Work out the finished part from the listing and answer in its coordinate system (mm). A direction names the side the tool comes from. Round coordinates to 2 decimals unless told otherwise and drop trailing zeros. Loops run counter-clockwise (first coordinate to the right, second up) from the corner with the lowest first, then second, coordinate; pieces in that order, holes last. Notation, with made-up numbers: (17, 53.5) - (74, 53.5) arc R20 ccw to (74, 83.5) - close; hole circle Ø5 at (-19.5, 22). An arc over 180 degrees is marked (long way). Return JSON: item names as keys, results as strings.
Autodesk Inventor part; units mm, degrees
ref_plane "YZ Plane" through (0, 0, 0) normal (1, 0, 0) x (0, 1, 0)
ref_plane "XZ Plane" through (0, 0, 0) normal (0, 1, 0) x (-1, 0, 0)
ref_plane "XY Plane" through (0, 0, 0) normal (0, 0, 1) x (1, 0, 0)
sketch "スケッチ1" plane through (0, 0, 0) normal (0, 0, 1) x (1, 0, 0)
  circle A0 centre (0, 0) radius 27.25
  line L0 (17.5, 17.5) -> (-17.5, 17.5)
  line L1 (-17.5, 17.5) -> (-17.5, -17.5)
  line L2 (-17.5, -17.5) -> (17.5, -17.5)
  line L3 (17.5, -17.5) -> (17.5, 17.5)
  line L4 (17.5, 17.5) -> (-17.5, -17.5) construction
  line L5 (-17.5, 17.5) -> (17.5, -17.5) construction
  line L6 (1, 17.5) -> (-1, 17.5)
  line L7 (-1, 17.5) -> (-1, -17.5)
  line L8 (-1, -17.5) -> (1, -17.5)
  line L9 (1, -17.5) -> (1, 17.5)
  line L10 (1, 17.5) -> (-1, -17.5) construction
  line L11 (-1, 17.5) -> (1, -17.5) construction
  point P0 (1, -17.5)
  point P1 (1, 17.5)
  point P2 (-1, 17.5)
  point P3 (-1, -17.5)
  dimension "d0" = 54.5
  dimension "d6" = 35
  dimension "d107" = 2
  dimension "d108" = 35
extrude "押し出し1" add sketch "スケッチ1" against normal blind 3 contours A0 | L9 L2 L7 L0
sketch "スケッチ2" plane through (0, 0, 0) normal (0, 0, 1) x (1, 0, 0)
  line L0 (0, 42.4511) -> (0, -37.5489)
  line L1 (38.0038, 0) -> (-41.9962, 0)
  line L2 (27.25, 42.0143) -> (27.25, -37.9857)
  circle A0 centre (0, 0) radius 27.25
  line L3 (17.5, 17.5) -> (17.5, -17.5)
  line L4 (19.25, 25) -> (27.25, 25)
  line L5 (27.25, 25) -> (27.25, -25)
  line L6 (27.25, -25) -> (19.25, -25)
  line L7 (19.25, -25) -> (19.25, 25)
  line L8 (19.25, 25) -> (27.25, -25) construction
  line L9 (27.25, 25) -> (19.25, -25) construction
  point P0 (17.5, 0)
  point P1 (23.25, 0)
  point P2 (19.25, 0)
  point P3 (27.25, 0)
  dimension "d13" = 9.75
  dimension "d14" = 8
  dimension "d15" = 50
  dimension "d19" = 54.5
  dimension "d110" = 1.75
extrude "押し出し2" cut sketch "スケッチ2" against normal blind 10 contours L7 L4 L2 A0 | A0 L1 L7 picked at (20.3822, 11.481)
mirror "ミラー1" about plane through (0, 0, 0) normal (1, 0, 0) of "押し出し2"
sketch "スケッチ8" plane through (0, 0, 0) normal (0, 0, 1) x (1, 0, 0)
  circle A0 centre (0, 0) radius 22.375
  circle A1 centre (0, 0) radius 27.25
  line L0 (0, 31.1603) -> (0, -30.8706)
  point P0 (0, 0)
  point P1 (0, 22.375)
  point P2 (0, -22.375)
  dimension "d112" = 44.75
  dimension "d113" = 54.5
hole "穴5" at (0, 22.375, 0) at (0, -22.375, 0) direction (0, 0, -1) diameter 6.6 end through all
properties part number "Part3_A_Y" material "鋼、軟鋼"
1) Section A-A (x = 0) is taken. Give the vertices of the cut face in (y, z) (3 decimals).
Verdict:
{"outline": "(-27.25, -3) - (-25.675, -3) - (-25.675, 0) - (-27.25, 0) - close; (-19.075, -3) - (19.075, -3) - (19.075, 0) - (-19.075, 0) - close; (25.675, -3) - (27.25, -3) - (27.25, 0) - (25.675, 0) - close"}
2) Section D-D (x = 8) is taken. Give the vertices of the cut face in (y, z).
Verdict:
{"outline": "(-26.05, -3) - (-17.5, -3) - (-17.5, 0) - (-26.05, 0) - close; (17.5, -3) - (26.05, -3) - (26.05, 0) - (17.5, 0) - close"}
3) A tool of negligible diameter and unlimited length cuts with its end or side. For faces 1 (the flat face through (9, 17.5, -1)), 2 (the flat face through (-23, 0, -1)), 3 (the flat face through (23, 0, -1)), from which of +Z, -Z, +X, -X, +Y, -Y can it reach the whole face along a straight path? Write none if from no direction.
Verdict:
{"face 1": "+Z, -Z", "face 2": "+Z, -Z, -X, +Y", "face 3": "+Z, -Z, +X, +Y"}
4) Determine the mould class of faces 4 (the flat face through (-1, 0, -1)), 5 (the cylindrical face through (-0.599, -27.243, -1.479)), 6 (the flat face through (0, 0, -3)) for opening direction Y: pulls with the +Y half, pulls with the -Y half, needs draft (parallel to the pull), parting line crosses it, or undercut.
Verdict:
{"face 4": "undercut", "face 5": "pulls with the -Y half", "face 6": "needs draft"}
5) Find the intervals of material crossed by L1, parallel to X at y = 6, z = -0.5; L2, parallel to Y at x = 0, z = -1.3 (3 decimals); L3, parallel to X at y = -10, z = -2.75, in increasing order.
Verdict:
{"L1": "x = -19.25 to -17.5, -1 to 1, 17.5 to 19.25", "L2": "y = -27.25 to -25.675, -19.075 to 19.075, 25.675 to 27.25", "L3": "x = -25.35 to -17.5, -1 to 1, 17.5 to 25.35"}
6) Section C-C (y = -12) is taken. Give the vertices of the cut face in (x, z).
Verdict:
{"outline": "(-24.47, -3) - (-17.5, -3) - (-17.5, 0) - (-24.47, 0) - close; (-1, -3) - (1, -3) - (1, 0) - (-1, 0) - close; (17.5, -3) - (24.47, -3) - (24.47, 0) - (17.5, 0) - close"}
7) Section B-B (z = -1.2) is taken. Give the vertices of the cut face in (x, y) (3 decimals), and give its area (3 significant figures).
Verdict:
{"outline": "(-27.25, 0) arc R27.25 ccw to (27.25, 0) - (19.25, 0) - (19.25, 19.287) arc R27.25 ccw to (-19.25, 19.287) - (-19.25, 0) - close; hole (-17.5, -17.5) - (-1, -17.5) - (-1, 17.5) - (-17.5, 17.5) - close; hole circle Ø6.6 at (0, -22.375); hole circle Ø6.6 at (0, 22.375); hole (1, -17.5) - (17.5, -17.5) - (17.5, 17.5) - (1, 17.5) - close", "area": "897 mm2"}
8) Flat-ended cylindrical pins translate along their axes: pin 1 (4 mm diameter, centred on x = 0, y = 22.375, fed in from -Z); pin 2 (1.5 mm diameter, centred on x = -23.5, z = -2, fed in from +Y); pin 3 (1 mm diameter, centred on y = 12.5, z = -2.5, fed in from -X); pin 4 (1.5 mm diameter, centred on y = 10.5, z = -2, fed in from +X). Find the tip coordinate at first contact, or state that the pin passes through.
Verdict:
{"pin 1": "passes through", "pin 2": "stops at y = 0", "pin 3": "stops at x = -19.25", "pin 4": "stops at x = 19.25"}
